```python
from build123d import *

# Parameters (mm, degrees)
Y_KSEKLIK_EKSTR_ZYON1_DEPTH = 10
IZIM2_R                     = 8
Y_KSEKLIK_EKSTR_ZYON2_DEPTH = 68
IZIM3_OUTSIDE_W             = 82.878
IZIM3_OUTSIDE_H             = 79.01
IZIM3_OUTSIDE_R             = 12.5
KES_EKSTR_ZYON2_DEPTH       = 10
KES_EKSTR_ZYON2_DRAFT       = -60


with BuildPart() as part:
    # Çizim1 → Yükseklik-Ekstrüzyon1 (new body)
    with BuildSketch(Plane.XY):
        Polygon((14.43375673, 0), (7.216878365, 12.5), (-7.216878365, 12.5), (-14.43375673, 0), (-7.216878365, -12.5), (7.216878365, -12.5), align=None)
    extrude(amount=Y_KSEKLIK_EKSTR_ZYON1_DEPTH)

    # Çizim2 → Yükseklik-Ekstrüzyon2 (add)
    with BuildSketch(Plane(origin=(0, 0, 0), x_dir=(-1, 0, 0), z_dir=(0, 0, -1))):
        Circle(IZIM2_R)
    extrude(amount=Y_KSEKLIK_EKSTR_ZYON2_DEPTH)


with BuildPart() as kes_ekstr_zyon2_tool:
    # Çizim3 outside → Kes-Ekstrüzyon2 (with draft: the straight prism first)
    with BuildSketch(Plane.XY.offset(10)):
        Rectangle(IZIM3_OUTSIDE_W, IZIM3_OUTSIDE_H)
        Circle(IZIM3_OUTSIDE_R, mode=Mode.SUBTRACT)
    extrude(amount=-KES_EKSTR_ZYON2_DEPTH)
    # Kes-Ekstrüzyon2: the draft: its side faces are tilted about the plane it starts from
    kes_ekstr_zyon2_sides = [kes_ekstr_zyon2_tool.faces().sort_by_distance(p)[0] for p in [
        (0, -39.505, 5),
        (41.439, 0, 5),
        (0, 39.505, 5),
        (-41.439, 0, 5),
        (-12.5, 0, 5),
    ]]
    draft(kes_ekstr_zyon2_sides, Plane.XY.offset(10), KES_EKSTR_ZYON2_DRAFT)


with BuildPart() as part_1:
    add(part.part)

    # Kes-Ekstrüzyon2: cut by kes_ekstr_zyon2_tool
    add(kes_ekstr_zyon2_tool.part, mode=Mode.SUBTRACT)


solid = part_1.part
```
Check sheet for the modelled part. Datum: model origin and axes. Units: mm. A direction names the side the tool comes from. Round coordinates to 2 decimals unless told otherwise and drop trailing zeros. Write each loop counter-clockwise with the first axis right and the second up, starting at its lowest first coordinate (ties: lowest second). Pieces come first, ordered by that corner, then holes. Notation, with made-up numbers: M 58.5,-29 L 82.5,-29 A28 cw 82.5,-2 Z; hole C 3,40 d2. An arc over 180 degrees is marked long. Write item = value, one per line. Start each with the question number.
1. Gauge pin test, flat ends, axial feed: pin 1 (10 mm diameter, centred on x = -6, z = -60, fed in from +Y); pin 2 (1.5 mm diameter, centred on x = -6, z = -19.5, fed in from +Y); pin 3 (1.5 mm diameter, centred on y = 3.5, z = -33, fed in from -X). Record the tip position at first contact, or that the pin passes through.
2. Tool access check on faces 1 (the flat face through (6.2, -5.4, 0)), 2 (the conical face through (-6.453, 11.24, 9.734)). Record the directions out of +Z, -Z, +X, -X, +Y, -Y that give a thin tool (end or side, any length) a straight path to the whole face; none if there is none.
3. Scan lines: line 1 (Z direction, x = 1.75, y = 11); line 2 (X direction, y = -5, z = -30) (3 decimals); line 3 (X direction, y = -5.5, z = -10.5). Record each from-to range of solid material in increasing order. Write a range as [from, to].
4. Section check A-A, the plane z = -4.5. Record the cut outline in (x, y), then the cut area to 3 significant figures.
Results found:
q1.pin_1 = 7.94
q1.pin_2 = 6.04
q1.pin_3 = -7.51
q2.face_1 = -Z
q2.face_2 = +Z, -X, +Y
q3.line_1 = [0, 10]
q3.line_2 = [-6.245, 6.245]
q3.line_3 = [-5.81, 5.81]
q4.outline = C 0,0 d16
q4.area = 201 mm^2
